from build123d import *

# Parameters (mm, degrees)
F0_R     = 63.5
F1_DEPTH = 20.32
F2_R     = 63.5
F3_DEPTH = 2.54
F4_R     = 5.08


with BuildPart() as f1:
    # F0 (on Front) → F1 (new body)
    with BuildSketch(Plane.XZ):
        Circle(F0_R)
        with BuildLine():
            ThreePointArc((41.82162, 24.082768), (46.622628, 12.464274), (48.26, 0))
            ThreePointArc((48.26, 0), (47.413582, -8.998878), (44.90402, -17.682099))
            ThreePointArc((44.90402, -17.682099), (32.785149, -35.414144), (14.172777, -46.131985))
            ThreePointArc((14.172777, -46.131985), (-7.246687, -47.712819), (-27.230856, -39.843545))
            ThreePointArc((-27.230856, -39.843545), (-41.82162, -24.082768), (-48.129099, -3.552103))
            ThreePointArc((-48.129099, -3.552103), (-44.90402, 17.682099), (-32.785149, 35.414144))
            ThreePointArc((-32.785149, 35.414144), (-14.172777, 46.131985), (7.246687, 47.712819))
            ThreePointArc((7.246687, 47.712819), (27.230856, 39.843545), (41.82162, 24.082768))
        make_face(mode=Mode.SUBTRACT)
    extrude(amount=-F1_DEPTH)

    # F2 (on Front) → F3 (join)
    with BuildSketch(Plane.XZ):
        Circle(F2_R)
    extrude(amount=F3_DEPTH)

    # F4
    f4_edges = [f1.edges().sort_by_distance(p)[0] for p in [
        (-63.5, -2.54, 0),
        (-63.5, 20.32, 0),
        (63.5, 8.89, 0),
    ]]
    fillet(f4_edges, radius=F4_R)


solid = f1.part
Here's how the part is built. I have some questions about the finished solid (model axes, mm). A direction names the side the tool comes from. Coordinates: 2 decimals unless noted, no trailing zeros. Order: outer loops, then holes, each group sorted by start corner. A loop starts at its lowest first (then second) coordinate and runs counter-clockwise, first axis right, second up.
Item 1: I need wall thicknesses on line 1 (Y direction, x = -32.5, z = -35); line 2 (X direction, y = 1.5, z = 33); line 3 (X direction, y = 14.5, z = 32.5). Which ranges of each line are inside material? Lowest first, please.
Result sheet:
line 1: y = -2.54 to 0
line 2: x = -54.13 to -35.21, 35.21 to 54.13
line 3: x = -54.55 to -35.68, 35.68 to 54.55
Item 2: For faces 5 (the face through (47.437, 10.018, -8.874)), 6 (the face through (-1, -2.54, 1)), which set-ups out of +Z, -Z, +X, -X, +Y, -Y let a thin tool reach every point of the face, with its end or its side?
Result sheet:
face 5: +Y
face 6: +Z, -Z, +X, -X, -Y
Item 3: If we mould it in two halves opening along Z, with no side actions, what happens to faces 1 (the face through (46.58, 10.02, 12.63)), 2 (the face through (60.57, 8.8, 19.07)), 3 (the face through (8, 20.32, 48)), 4 (the face through (-1, 0, 1))? For each: +Z half, -Z half, draft (parallel to the pull), parting line (faces both ways), or undercut.
Result sheet:
face 1: undercut
face 2: parting line
face 3: draft
face 4: undercut
Item 4: For P1, Ø1, axis at x = 14.5, y = 10, coming from the -Z side; P2, Ø2, axis at y = 9, z = -3, coming from the -X side; P3, Ø3, axis at x = -16.5, z = -11, coming from the +Y side, each with a flat end and sliding along its axis, tell me the tip position at first contact or that it passes through.
Result sheet:
P1: stops at z = -61.94
P2: stops at x = -63.47
P3: stops at y = 0
Item 5: If we section it at A-A on y = 11: List the corners of the cut face in (x, z) for me.
Result sheet:
outline: circle Ø127 at (0, 0); hole (-48.13, -3.55) arc R48.26 ccw to (-27.23, -39.84) arc R48.26 ccw to (14.17, -46.13) arc R48.26 ccw to (44.9, -17.68) arc R48.26 ccw to (48.26, 0) arc R48.26 ccw to (41.82, 24.08) arc R48.26 ccw to (7.25, 47.71) arc R48.26 ccw to (-32.79, 35.41) arc R48.26 ccw to start
Item 6: If we section it at B-B on y = 18.5: List the corners of the cut face in (x, z) for me.
Result sheet:
outline: circle Ø124.63 at (0, 0); hole (-48.13, -3.55) arc R48.26 ccw to (-27.23, -39.84) arc R48.26 ccw to (14.17, -46.13) arc R48.26 ccw to (44.9, -17.68) arc R48.26 ccw to (48.26, 0) arc R48.26 ccw to (41.82, 24.08) arc R48.26 ccw to (7.25, 47.71) arc R48.26 ccw to (-32.79, 35.41) arc R48.26 ccw to start
